```python
from build123d import *

# Parameters (mm, degrees)
SKETCH1_W           = 210
SKETCH1_H           = 20
BOSS_EXTRUDE1_DEPTH = 15
SKETCH2_W           = 210
SKETCH2_H           = 10
CUT_EXTRUDE1_DEPTH  = 10
SKETCH3_R           = 1.8
CUT_EXTRUDE2_DEPTH  = 6
SKETCH5_R           = 3.5
CUT_EXTRUDE3_DEPTH  = 3.6
SKETCH6_W           = 210
SKETCH6_H           = 10
CUT_EXTRUDE4_DEPTH  = 0.6
SKETCH7_W           = 210
SKETCH7_H           = 10
CUT_EXTRUDE5_DEPTH  = 0.6


with BuildPart() as part:
    # Sketch1 → Boss-Extrude1 (new body)
    with BuildSketch(Plane(origin=(0, 0, 0), x_dir=(1, 0, 0), z_dir=(0, 1, 0))):
        with Locations((105, 10)):
            Rectangle(SKETCH1_W, SKETCH1_H)
    extrude(amount=BOSS_EXTRUDE1_DEPTH)

    # Sketch2 → Cut-Extrude1 (cut)
    with BuildSketch(Plane(origin=(0, 15, 0), x_dir=(1, 0, 0), z_dir=(0, 1, 0))):
        with Locations((105, 10)):
            Rectangle(SKETCH2_W, SKETCH2_H)
    extrude(amount=-CUT_EXTRUDE1_DEPTH, mode=Mode.SUBTRACT)

    # Sketch3 → Cut-Extrude2 (cut, through all)
    with BuildSketch(Plane(origin=(0, 5, 0), x_dir=(1, 0, 0), z_dir=(0, 1, 0))):
        with Locations((25, 10)):
            Circle(SKETCH3_R)
    cut_extrude2 = extrude(amount=-CUT_EXTRUDE2_DEPTH, mode=Mode.SUBTRACT)

    # Sketch5 → Cut-Extrude3 (cut)
    with BuildSketch(Plane(origin=(0, 5, 0), x_dir=(1, 0, 0), z_dir=(0, 1, 0))):
        with Locations((25, 10)):
            Circle(SKETCH5_R)
    cut_extrude3 = extrude(amount=-CUT_EXTRUDE3_DEPTH, mode=Mode.SUBTRACT)

    # Mirror2: Cut-Extrude2, Cut-Extrude3 across plane
    add(cut_extrude2.mirror(Plane(origin=(58.611943839, 0, 0), x_dir=(0, 0, 1), z_dir=(1, 0, 0))), mode=Mode.SUBTRACT)
    add(cut_extrude3.mirror(Plane(origin=(58.611943839, 0, 0), x_dir=(0, 0, 1), z_dir=(1, 0, 0))), mode=Mode.SUBTRACT)

    # Sketch6 → Cut-Extrude4 (cut)
    with BuildSketch(Plane.XY.offset(-15)):
        with Locations((105, 10)):
            Rectangle(SKETCH6_W, SKETCH6_H)
    extrude(amount=-CUT_EXTRUDE4_DEPTH, mode=Mode.SUBTRACT)

    # Sketch7 → Cut-Extrude5 (cut)
    with BuildSketch(Plane(origin=(0, 0, -5), x_dir=(-1, 0, 0), z_dir=(0, 0, -1))):
        with Locations((-105, 10)):
            Rectangle(SKETCH7_W, SKETCH7_H)
    extrude(amount=-CUT_EXTRUDE5_DEPTH, mode=Mode.SUBTRACT)


solid = part.part
```
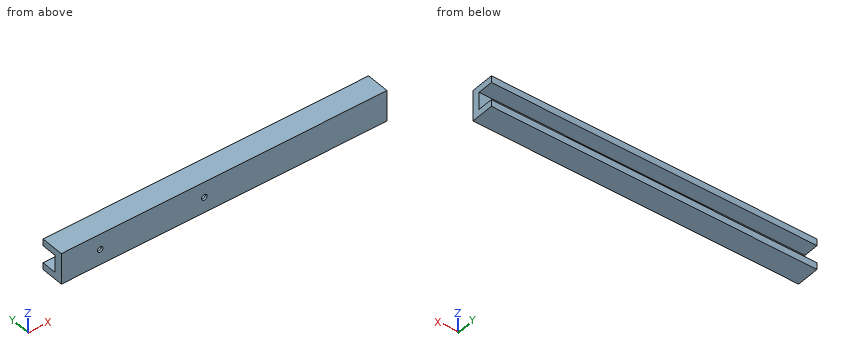
Design review of the part built by this model. Coordinates are the model's own, in mm. Coordinates: 2 decimals unless noted, no trailing zeros. Loops run counter-clockwise (first coordinate to the right, second up) from the corner with the lowest first, then second, coordinate; pieces in that order, holes last. Notation, with made-up numbers: (20.5, 84) -> (26.5, 84) arc R10 ccw to (26.5, 103) -> close; hole circle Ø9 at (51.5, -8.75). An arc over 180 degrees is marked (long way). Answer as a JSON object with one key per item and string values.
Q1. Take a section at A-A on y = 8.75. Give the boundary of the cut face in (x, z), plus the area to 3 significant figures.
Answer block:
{"outline": "(0, -20) -> (210, -20) -> (210, -15.6) -> (0, -15.6) -> close; (0, -4.4) -> (210, -4.4) -> (210, 0) -> (0, 0) -> close", "area": "1,850 mm^2"}
Q2. Take a section at D-D on x = 129. Give the boundary of the cut face in (y, z).
Answer block:
{"outline": "(0, -20) -> (15, -20) -> (15, -15.6) -> (5, -15.6) -> (5, -4.4) -> (15, -4.4) -> (15, 0) -> (0, 0) -> close"}
Q3. Take a section at B-B on z = -10. Give the boundary of the cut face in (x, y).
Answer block:
{"outline": "(0, 0) -> (23.2, 0) -> (23.2, 1.4) -> (21.5, 1.4) -> (21.5, 5) -> (0, 5) -> close; (26.8, 0) -> (90.42, 0) -> (90.42, 1.4) -> (88.72, 1.4) -> (88.72, 5) -> (28.5, 5) -> (28.5, 1.4) -> (26.8, 1.4) -> close; (94.02, 0) -> (210, 0) -> (210, 5) -> (95.72, 5) -> (95.72, 1.4) -> (94.02, 1.4) -> close"}
Q4. Take a section at C-C on x = 25. Give the boundary of the cut face in (y, z), plus the area to 3 significant figures.
Answer block:
{"outline": "(0, -20) -> (15, -20) -> (15, -15.6) -> (5, -15.6) -> (5, -13.5) -> (1.4, -13.5) -> (1.4, -11.8) -> (0, -11.8) -> close; (0, -8.2) -> (1.4, -8.2) -> (1.4, -6.5) -> (5, -6.5) -> (5, -4.4) -> (15, -4.4) -> (15, 0) -> (0, 0) -> close", "area": "158 mm^2"}
Q5. Clearance check with flat-ended pins moving along their axes: pin 1 Ø2 at (x, z) = (25, -11.5) entering from +Y; pin 2 Ø8 at (x, z) = (25, -10) entering from +Y. State where each tip first meets the part, or that it passes through.
Answer block:
{"pin 1": "stops at y = 1.4", "pin 2": "stops at y = 5"}
Q6. To check wall thickness, follow L1, parallel to X at y = 3, z = -10; L2, parallel to Z at x = 127.5, y = 11.5; L3, parallel to Z at x = 25, y = 0.8. State the ranges of each line that lie inside material, in increasing order.
Answer block:
{"L1": "x = 0 to 21.5, 28.5 to 88.72, 95.72 to 210", "L2": "z = -20 to -15.6, -4.4 to 0", "L3": "z = -20 to -11.8, -8.2 to 0"}
